Answer from the drawing. Dimensions are ordinates in mm from the lowest x, y and z of the part. Coordinates: 2 decimals unless noted, no trailing zeros. Loops run counter-clockwise (first coordinate to the right, second up) from the corner with the lowest first, then second, coordinate; pieces in that order, holes last.
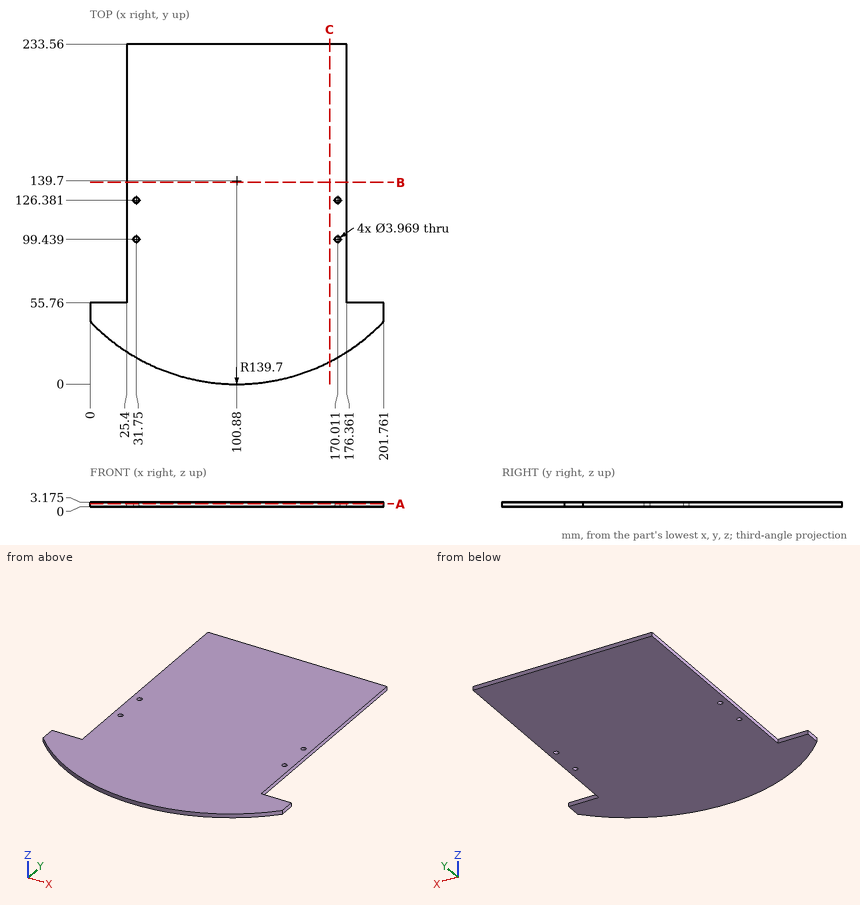
Item 1: Find the intervals of material crossed by line 1 along Y through (x, z) = (30, 1.8) (1 decimal); line 2 along Y through (x, z) = (31.75, 1.3) (1 decimal); line 3 along X through (y, z) = (150.5, 1.15), in increasing order.
Numbers:
line 1: y = 19.3 to 98.5, 100.4 to 125.4, 127.3 to 233.6
line 2: y = 18.3 to 97.5, 101.4 to 124.4, 128.4 to 233.6
line 3: x = 25.4 to 176.36
Item 2: A cutting plane is placed at A-A on z = 2.05. Give the number of separate pieces and of enclosed holes in the cut face, then the cut area to 3 significant figures.
Numbers:
separate pieces: 1
enclosed holes: 4
area: 35,400 mm2
Item 3: A cutting plane is placed at B-B on y = 138.5. Determine the outline of the cut face in (x, z) (1 decimal).
Numbers:
outline: (25.4, 0) - (176.4, 0) - (176.4, 3.2) - (25.4, 3.2) - close
Item 4: A cutting plane is placed at C-C on x = 164.5. Determine the outline of the cut face in (y, z) (1 decimal).
Numbers:
outline: (15.3, 0) - (233.6, 0) - (233.6, 3.2) - (15.3, 3.2) - close
Item 5: Given pin 1 (1 mm diameter, centred on x = 69, y = 99.5, fed in from -Z); pin 2 (1 mm diameter, centred on x = 187.5, z = 2.5, fed in from +Y); pin 3 (1 mm diameter, centred on y = 128.5, z = 2.5, fed in from +X); pin 4 (1 mm diameter, centred on y = 152.5, z = 1, fed in from -X), each flat-ended and moving along its own axis, determine where each tip first touches the part or whether it passes through.
Numbers:
pin 1: stops at z = 0
pin 2: stops at y = 55.76
pin 3: stops at x = 176.36
pin 4: stops at x = 25.4
